```python
from build123d import *

# Parameters (mm, degrees)
SKETCH027_W             = 40
SKETCH027_H             = 38
PAD018_DEPTH            = 3
SKETCH028_W             = 40
SKETCH028_H             = 3
PAD019_DEPTH            = 39
SKETCH029_R             = 1.5
SKETCH029_W             = 24
SKETCH029_H             = 25
POCKET009_DEPTH         = 5
POCKET010_DEPTH         = 5
PAD020_DEPTH            = 3
PAD021_DEPTH            = 3
FILLET012_R             = 8
BODY006_PLACEMENT_ANGLE = 180


with BuildPart() as part:
    # Sketch027 (on Face1 of Binder004) → Pad018 (new body)
    with BuildSketch(Plane(origin=(0, 0, 3.2), x_dir=(1, 0, 0), z_dir=(0, 0, -1))):
        with Locations((-83.6396103068, 84.6396103068)):
            Rectangle(SKETCH027_W, SKETCH027_H)
    extrude(amount=PAD018_DEPTH)

    # Sketch028 (on Face6 of Pad018) → Pad019 (join)
    with BuildSketch(Plane(origin=(0, 0, 0.2), x_dir=(1, 0, 0), z_dir=(0, 0, -1))):
        with Locations((-83.6396103068, 67.1396103068)):
            Rectangle(SKETCH028_W, SKETCH028_H)
    extrude(amount=PAD019_DEPTH)

    # Sketch029 (on Face7 of Pad019) → Pocket009 (cut)
    with BuildSketch(Plane(origin=(0, -65.6396103068, 0), x_dir=(-1, 0, 0), z_dir=(0, 1, 0))):
        with Locations((-92.5127987438, -33.2127134049)):
            Circle(SKETCH029_R)
        with Locations((-73.1038955613, -33.2)):
            Circle(SKETCH029_R)
        with Locations((83.6396103068, -14.3)):
            Rectangle(SKETCH029_W, SKETCH029_H)
    extrude(amount=-POCKET009_DEPTH, mode=Mode.SUBTRACT)

    # Sketch030 (on Face4 of Pocket009) → Pocket010 (cut)
    with BuildSketch(Plane.XY.offset(3.2)):
        Polygon((-91.417785, -87.175144), (-95.660426, -91.417785), (-91.417785, -95.660426), (-87.175144, -91.417785), align=None)
        Polygon((-80.104076, -91.417785), (-75.861436, -87.175144), (-71.618795, -91.417785), (-75.861436, -95.660426), align=None)
        Polygon((-91.417785, -80.104076), (-87.175144, -75.861436), (-91.417785, -71.618795), (-95.660426, -75.861436), align=None)
        Polygon((-80.104076, -75.861436), (-75.861436, -80.104076), (-71.618795, -75.861436), (-75.861436, -71.618795), align=None)
    extrude(amount=-POCKET010_DEPTH, mode=Mode.SUBTRACT)

    # Sketch031 (on Face3 of Pocket010) → Pad020 (join)
    with BuildSketch(Plane(origin=(-103.6396103068, 0, 0), x_dir=(0, -1, 0), z_dir=(-1, 0, 0))):
        Polygon((88.6396103068, 0.2), (68.6396103068, -19.8), (68.6396103068, 0.2), align=None)
    extrude(amount=-PAD020_DEPTH)

    # Sketch032 (on Face2 of Pad020) → Pad021 (join)
    with BuildSketch(Plane.YZ.offset(-63.6396103068)):
        Polygon((-88.6396103068, 0.2), (-68.6396103068, 0.2), (-68.6396103068, -19.8), align=None)
    extrude(amount=-PAD021_DEPTH)

    # Fillet012
    fillet012_edges = [part.edges().sort_by_distance(p)[0] for p in [
        (-103.63961, -103.63961, 1.7),
    ]]
    fillet(fillet012_edges, radius=FILLET012_R)


with BuildPart() as part_1:
    # Body006 placement: moved
    add(part.part.rotate(Axis((0, 0, 0), (0, 0, 1)), BODY006_PLACEMENT_ANGLE))


solid = part_1.part
```
Geometry check sheet. Reference: the model listing, model coordinates, mm. A direction names the side the tool comes from. Coordinates: 2 decimals unless noted, no trailing zeros. Loops run counter-clockwise (first coordinate to the right, second up) from the corner with the lowest first, then second, coordinate; pieces in that order, holes last. Notation, with made-up numbers: (6.5, 43.5) -> (49.5, 43.5) arc R14 ccw to (49.5, 57.5) -> close; hole circle Ø3 at (19.25, 86). An arc over 180 degrees is marked (long way). Put each result on its own line as item: value.
1) Tool access check on faces 1 (the flat face through (83, 67, -1.8)), 2 (the flat face through (84, 86, 0.2)), 3 (the flat face through (73.71, 73.77, 1.72)). Record the directions out of +Z, -Z, +X, -X, +Y, -Y that give a thin tool (end or side, any length) a straight path to the whole face; none if there is none.
Result set:
face 1: +Y, -Y
face 2: -Z, +Y
face 3: +Z, -Z
2) Cross-section at B-B on z = -21.5. Record the boundary of the cut face in (x, y), plus the area to 3 significant figures.
Result set:
outline: (63.64, 65.64) -> (71.64, 65.64) -> (71.64, 68.64) -> (63.64, 68.64) -> close; (95.64, 65.64) -> (103.64, 65.64) -> (103.64, 68.64) -> (95.64, 68.64) -> close
area: 48.0 mm^2
3) Thickness scan on line 1 (X direction, y = 78, z = -4); line 2 (Y direction, x = 78, z = 0.5); line 3 (Y direction, x = 69, z = -25). Record the ranges inside material, lowest first.
Result set:
line 1: x = 63.64 to 66.64, 100.64 to 103.64
line 2: y = 65.64 to 73.76, 77.97 to 89.31, 93.52 to 103.64
line 3: y = 65.64 to 68.64
4) Cross-section at A-A on x = 84. Record the boundary of the cut face in (y, z).
Result set:
outline: (65.64, -38.8) -> (68.64, -38.8) -> (68.64, -26.8) -> (65.64, -26.8) -> close; (65.64, -1.8) -> (68.64, -1.8) -> (68.64, 0.2) -> (103.64, 0.2) -> (103.64, 3.2) -> (65.64, 3.2) -> close
5) Release check for a two-part mould opening along X. For faces 4 (the flat face through (103.64, 74, -8)), 5 (the flat face through (89.267, 89.326, 1.721)), 6 (the flat face through (84, 85, 3.2)) record: released by +X, released by -X, zero draft, split by the parting line, or undercut.
Result set:
face 4: released by +X
face 5: undercut
face 6: zero draft
6) Cross-section at D-D on y = 73.5. Record the boundary of the cut face in (x, z), plus the area to 3 significant figures.
Result set:
outline: (63.64, -14.94) -> (66.64, -14.94) -> (66.64, 0.2) -> (73.98, 0.2) -> (73.98, 3.2) -> (63.64, 3.2) -> close; (77.74, 0.2) -> (89.54, 0.2) -> (89.54, 3.2) -> (77.74, 3.2) -> close; (93.3, 0.2) -> (100.64, 0.2) -> (100.64, -14.94) -> (103.64, -14.94) -> (103.64, 3.2) -> (93.3, 3.2) -> close
area: 188 mm^2
7) Cross-section at C-C on x = 93.5. Record the boundary of the cut face in (y, z), plus the area to 3 significant figures.
Result set:
outline: (65.64, -38.8) -> (68.64, -38.8) -> (68.64, -26.8) -> (65.64, -26.8) -> close; (65.64, -1.8) -> (68.64, -1.8) -> (68.64, 0.2) -> (73.7, 0.2) -> (73.7, 3.2) -> (65.64, 3.2) -> close; (78.02, 0.2) -> (89.26, 0.2) -> (89.26, 3.2) -> (78.02, 3.2) -> close; (93.58, 0.2) -> (103.64, 0.2) -> (103.64, 3.2) -> (93.58, 3.2) -> close
area: 130 mm^2
8) Gauge pin test, flat ends, axial feed: pin 1 Ø1.5 at (x, z) = (98, -18.5) entering from +Y; pin 2 Ø10.5 at (x, y) = (81, 81) entering from -Z; pin 3 Ø12 at (y, z) = (76, -18) entering from -X. Record the tip position at first contact, or that the pin passes through.
Result set:
pin 1: stops at y = 68.64
pin 2: stops at z = 0.2
pin 3: stops at x = 63.64
